Autodesk Inventor part; units mm, degrees
ref_plane "YZ Plane" through (0, 0, 0) normal (1, 0, 0) x (0, 1, 0)
ref_plane "XZ Plane" through (0, 0, 0) normal (0, 1, 0) x (-1, 0, 0)
ref_plane "XY Plane" through (0, 0, 0) normal (0, 0, 1) x (1, 0, 0)
sketch "Skizze1" plane through (0, 0, 0) normal (0, 0, 1) x (1, 0, 0)
  circle A0 centre (-10.5, 14.452) radius 10.5
  circle A1 centre (0, 0) radius 17.8637 construction
  circle A2 centre (10.5, 14.452) radius 10.5
  circle A3 centre (16.9894, -5.5202) radius 10.5
  circle A4 centre (0, -17.8637) radius 10.5
  circle A5 centre (-16.9894, -5.5202) radius 10.5
  arc A6 (-13.7447, 4.4659) -> (0, 14.452) centre (-10.5, 14.452) ccw
  arc A7 (0, 14.452) -> (13.7447, 4.4659) centre (10.5, 14.452) ccw
  arc A8 (13.7447, 4.4659) -> (8.4947, -11.6919) centre (16.9894, -5.5202) ccw
  arc A9 (8.4947, -11.6919) -> (-8.4947, -11.6919) centre (0, -17.8637) ccw
  arc A10 (-8.4947, -11.6919) -> (-13.7447, 4.4659) centre (-16.9894, -5.5202) ccw
  dimension "d0" = 21
  dimension "d1" = 10.5
extrude "Extrusion1" add sketch "Skizze1" along normal blind 50 contours A2 A3 A4 A5 A0
fillet "Rundung1" radius 0.5 5 edges at (0, 14.452, 25) (13.7447, 4.4659, 25) (-13.7447, 4.4659, 25) (-8.4947, -11.6919, 25) (8.4947, -11.6919, 25)
sketch "Skizze2" plane through (0, 0, 50) normal (0, 0, 1) x (1, 0, 0)
  arc A0 (6.269, -9.4405) -> (7.0412, -8.8794) centre (6.5675, -9.0394) ccw
  arc A1 (10.9157, 3.0449) -> (7.0412, -8.8794) centre (16.9894, -5.5202) ccw
  arc A2 (10.9157, 3.0449) -> (10.6207, 3.9527) centre (10.6264, 3.4527) ccw
  arc A3 (0.4773, 11.3223) -> (10.6207, 3.9527) centre (10.5, 14.452) ccw
  arc A4 (0.4773, 11.3223) -> (-0.4773, 11.3223) centre (0, 11.1733) ccw
  arc A5 (-10.6207, 3.9527) -> (-0.4773, 11.3223) centre (-10.5, 14.452) ccw
  arc A6 (-10.6207, 3.9527) -> (-10.9157, 3.0449) centre (-10.6264, 3.4527) ccw
  arc A7 (-7.0412, -8.8794) -> (-10.9157, 3.0449) centre (-16.9894, -5.5202) ccw
  arc A8 (-7.0412, -8.8794) -> (-6.269, -9.4405) centre (-6.5675, -9.0394) ccw
  arc A9 (6.269, -9.4405) -> (-6.269, -9.4405) centre (0, -17.8637) ccw
  arc A10 (8.8359, 2.871) -> (5.4609, -7.5163) centre (16.9894, -5.5202) ccw
  arc A11 (5.4609, -7.5163) -> (-5.4609, -7.5163) centre (0, -17.8637) ccw
  arc A12 (-5.4609, -7.5163) -> (-8.8359, 2.871) centre (-16.9894, -5.5202) ccw
  arc A13 (-8.8359, 2.871) -> (0, 9.2906) centre (-10.5, 14.452) ccw
  arc A14 (0, 9.2906) -> (8.8359, 2.871) centre (10.5, 14.452) ccw
  point P0 (0, 0)
  dimension "d5" = 1.2
extrude "Extrusion2" cut sketch "Skizze2" against normal through all contours A10 A11 A12 A13 A14
equation "\"G_L\" = 0"
equation "\"G_H\" = 0"
equation "\"G_B\" = 0"
properties part number "21700_stern" material "GEDA Stahl"
Verification items for the finished model (mm, model axes). Coordinates: 2 decimals unless noted, no trailing zeros. Write each loop counter-clockwise with the first axis right and the second up, starting at its lowest first coordinate (ties: lowest second). Pieces come first, ordered by that corner, then holes. Notation, with made-up numbers: (-30, 26) -> (-12, 26) arc R15 ccw to (-12, 54) -> close; hole circle Ø3 at (30, 74). An arc over 180 degrees is marked (long way). One line per item, written item: value. Start each with the question number.
Q1. Cross-section at A-A on x = -2.5. Enter the section's corners in (y, z).
Q2. Go/stop test with flat-tipped pins: P1, Ø3, axis at x = -4.5, z = 26, coming from the +Y side; P2, Ø1, axis at y = 2.5, z = 23, coming from the +X side; P3, Ø2, axis at y = 9.5, z = 30, coming from the +X side. Record where each tip stops, or that it passes through.
Q3. Thickness scan on L1, parallel to X at y = -7, z = 31.5; L2, parallel to X at y = 0, z = 43; L3, parallel to Y at x = -7.5, z = 33. Record the ranges inside material, lowest first. Write a range as from..to.
Q4. Cross-section at C-C on y = 10.75. Enter the section's corners in (x, z), and give its area (3 significant figures).
Q5. Mould release check, pull along X, two halves, no side actions. Record for faces 1 (the cylindrical face through (6.975, -2.365, 24.65)), 2 (the cylindrical face through (-5.838, -1.98, 25.35)), 3 (the flat face through (-6, -2, 50)), 4 (the cylindrical face through (-7.03, -2.19, 24.65)): pulls with the +X half, pulls with the -X half, needs draft (parallel to the pull), parting line crosses it, or undercut.
Q6. Cross-section at B-B on y = -3.25. Enter the section's corners in (x, z).
Checked values:
1. outline: (-7.67, 0) -> (-6.43, 0) -> (-6.43, 50) -> (-7.67, 50) -> close; (5.91, 0) -> (7.65, 0) -> (7.65, 50) -> (5.91, 50) -> close
2. P1: stops at y = 7.1
2. P2: stops at x = 10.85
2. P3: stops at x = 1.85
3. L1: x = -6.59..-5.38, -4.34..4.34, 5.38..6.59
3. L2: x = -8.06..-6.67, 6.67..8.06
3. L3: y = -1.03..1.32, 3.14..4.39
4. outline: (-0.67, 0) -> (0.67, 0) -> (0.67, 50) -> (-0.67, 50) -> close
4. area: 67.4 mm²
5. face 1: pulls with the +X half
5. face 2: undercut
5. face 3: needs draft
5. face 4: pulls with the -X half
6. outline: (-6.74, 0) -> (-5.51, 0) -> (-5.51, 50) -> (-6.74, 50) -> close; (5.51, 0) -> (6.74, 0) -> (6.74, 50) -> (5.51, 50) -> close
